Autodesk Inventor part; units mm, degrees
ref_plane "YZ Plane" through (0, 0, 0) normal (1, 0, 0) x (0, 1, 0)
ref_plane "XZ Plane" through (0, 0, 0) normal (0, 1, 0) x (-1, 0, 0)
ref_plane "XY Plane" through (0, 0, 0) normal (0, 0, 1) x (1, 0, 0)
sketch "Sketch2" plane through (0, 0, 0) normal (0, 0, 1) x (1, 0, 0)
  line L0 (0, 0) -> (44.45, 0)
  line L1 (44.45, 0) -> (44.45, 50.8)
  line L2 (44.45, 50.8) -> (0, 50.8)
  line L3 (0, 50.8) -> (0, 0)
  dimension "d0" = 50.8
  dimension "d1" = 44.45
extrude "Extrusion1" add sketch "Sketch2" along normal blind 25.4
sketch "Sketch3" plane through (0, 0, 25.4) normal (0, 0, 1) x (1, 0, 0)
  line L0 (2.54, 2.54) -> (20.32, 2.54)
  line L1 (20.32, 2.54) -> (20.32, 48.26)
  line L2 (20.32, 48.26) -> (2.54, 48.26)
  line L3 (2.54, 48.26) -> (2.54, 2.54)
  line L4 (0, 0) -> (44.45, 0)
  line L5 (0, 50.8) -> (0, 0)
  line L6 (44.45, 50.8) -> (0, 50.8)
  line L7 (21.59, 2.54) -> (41.91, 2.54)
  line L8 (41.91, 2.54) -> (41.91, 48.26)
  line L9 (41.91, 48.26) -> (21.59, 48.26)
  line L10 (21.59, 48.26) -> (21.59, 2.54)
  line L11 (44.45, 0) -> (44.45, 50.8)
  dimension "d4" = 2.54
  dimension "d5" = 2.54
  dimension "d6" = 2.54
  dimension "d7" = 20.32
  dimension "d8" = 2.54
  dimension "d9" = 2.54
  dimension "d10" = 2.54
  dimension "d11" = 22.86
extrude "Extrusion2" cut sketch "Sketch3" against normal blind 20.32 contours L3 L2 L1 L0 | L10 L9 L8 L7
sketch "Sketch4" plane through (0, 0, 0) normal (0, 0, -1) x (-1, 0, 0)
  circle A0 centre (-12.7, 17.78) radius 8.89
  line L0 (0, 50.8) -> (0, 0)
  line L1 (0, 0) -> (-44.45, 0)
  dimension "d14" = 17.78
  dimension "d17" = 12.7
  dimension "d18" = 17.78
extrude "Extrusion3" cut sketch "Sketch4" against normal blind 3.175
sketch "Sketch5" plane through (0, 0, 0) normal (0, 0, -1) x (-1, 0, 0)
  point P0 (0, 0)
sketch "Sketch6" plane through (12.7, 17.78, 3.175) normal (0, 0, -1) x (-1, 0, 0)
  circle A0 centre (0, 0) radius 8.89
  line L0 (0, 0) -> (-5.08, 0)
  line L1 (-5.08, 0) -> (-5.08, 12.7)
  line L2 (-5.08, 12.7) -> (0, 12.7)
  line L3 (0, 12.7) -> (0, 0)
  line L4 (0, 0) -> (5.08, 0)
  line L5 (5.08, 0) -> (5.08, 12.7)
  line L6 (5.08, 12.7) -> (0, 12.7)
  line L7 (0, 12.7) -> (0, 0)
  point P0 (12.7, -17.78)
  dimension "d21" = 12.7
  dimension "d22" = 5.08
  dimension "d23" = 5.08
extrude "Extrusion4" cut sketch "Sketch6" along normal blind 5.08 contours L5 L4 L3 A0 | A0 L3 L6 L5 | L1 L2 L3 A0 | A0 L3 L0 L1
sketch "Sketch7" plane through (0, 0, 3.175) normal (0, 0, -1) x (-1, 0, 0)
  point P0 (0, 0)
sketch "Sketch8" plane through (0, 0, 3.175) normal (0, 0, -1) x (-1, 0, 0)
  line L0 (-7.62, 25.0756) -> (-7.62, 30.48)
  line L1 (-17.78, 30.48) -> (-7.62, 30.48)
  line L2 (-7.62, 30.48) -> (-7.62, 26.67)
  line L3 (-7.62, 26.67) -> (-17.78, 26.67)
  line L4 (-17.78, 26.67) -> (-17.78, 30.48)
  point P0 (0, 0)
  dimension "d26" = 3.81
extrude "Extrusion5" cut sketch "Sketch8" against normal blind 2.54
sketch "Sketch14" plane through (41.91, 2.54, 25.4) normal (-1, 0, 0) x (0, 0, 1)
  line L0 (0, 0) -> (-20.32, 0)
  line L1 (0, 45.72) -> (-20.32, 45.72)
  line L2 (-12.7, 45.72) -> (-12.7, 43.18)
  line L3 (-12.7, 43.18) -> (-15.24, 45.72)
  line L4 (-12.7, 0) -> (-12.7, 2.54)
  line L5 (-12.7, 2.54) -> (-15.24, 0)
  point P0 (-25.4, -2.54)
  dimension "d52" = 45
  dimension "d53" = 2.54
  dimension "d54" = 2.54
  dimension "d55" = 45
  dimension "d56" = 5.08
  dimension "d57" = 5.08
extrude "Arduino Holder" add sketch "Sketch14" along normal blind 20.32
sketch "Sketch16" plane through (2.54, 2.54, 25.4) normal (0, 1, 0) x (1, 0, 0)
  line L0 (0, 12.7) -> (3.81, 12.7)
  line L1 (3.81, 12.7) -> (0, 16.51)
  line L2 (0, 0) -> (0, 20.32)
  line L3 (17.78, 5.08) -> (17.78, 20.32)
  line L4 (17.78, 16.51) -> (13.97, 12.7)
  line L5 (13.97, 12.7) -> (17.78, 12.7)
  line L6 (17.78, 20.32) -> (0, 20.32)
  point P0 (-2.54, 25.4)
  dimension "d60" = 45
  dimension "d61" = 3.81
  dimension "d62" = 3.81
  dimension "d64" = 45
  dimension "d144" = 7.62
  dimension "d145" = 7.62
extrude "Bluetooth Holder" add sketch "Sketch16" along normal blind 45.72
sketch "Sketch17" plane through (0, 0, 0) normal (-1, 0, 0) x (0, 0, 1)
  line L0 (0, 50.8) -> (25.4, 50.8)
  line L1 (0, 0) -> (5.08, 0)
  line L2 (5.08, 0) -> (5.08, 50.8)
  line L3 (5.08, 50.8) -> (0, 50.8)
  line L4 (0, 50.8) -> (0, 0)
  dimension "d68" = 5.08
extrude "Extrusion13" add sketch "Sketch17" along normal blind 5.08
sketch "Sketch18" plane through (0, 0, 5.08) normal (0, 0, 1) x (1, 0, 0)
  line L0 (0, 50.8) -> (0, 0)
  line L1 (0, 2.54) -> (-2.54, 2.54)
  line L2 (-2.54, 2.54) -> (-2.54, 48.26)
  line L3 (-2.54, 48.26) -> (0, 48.26)
  line L4 (0, 48.26) -> (0, 2.54)
  line L5 (0, 50.8) -> (-5.08, 50.8)
  line L6 (0, 0) -> (-5.08, 0)
  dimension "d71" = 2.54
  dimension "d72" = 2.54
  dimension "d73" = 2.54
extrude "Extrusion14" cut sketch "Sketch18" against normal blind 5.08
sketch "Sketch19" plane through (44.45, 0, 0) normal (1, 0, 0) x (0, 0, -1)
  line L0 (0, 50.8) -> (-25.4, 50.8)
  line L1 (0, 0) -> (-5.08, 0)
  line L2 (-5.08, 0) -> (-5.08, 50.8)
  line L3 (-5.08, 50.8) -> (0, 50.8)
  line L4 (0, 50.8) -> (0, 0)
  dimension "d76" = 5.08
extrude "Extrusion15" add sketch "Sketch19" along normal blind 5.08
sketch "Sketch21" plane through (44.45, 0, 5.08) normal (0, 0, 1) x (1, 0, 0)
  line L0 (0, 0) -> (0, 50.8)
  line L1 (0, 2.54) -> (2.54, 2.54)
  line L2 (2.54, 2.54) -> (2.54, 48.26)
  line L3 (2.54, 48.26) -> (0, 48.26)
  line L4 (0, 48.26) -> (0, 2.54)
  line L5 (0, 50.8) -> (5.08, 50.8)
  line L6 (0, 0) -> (5.08, 0)
  line L7 (5.08, 50.8) -> (5.08, 0)
  point P0 (-44.45, 0)
  dimension "d79" = 2.54
  dimension "d81" = 2.54
  dimension "d82" = 2.54
extrude "Extrusion16" cut sketch "Sketch21" against normal blind 5.08 contours L0 L3 L2 L1
sketch "Sketch28" plane through (0, 0, 25.4) normal (-1, 0, 0) x (0, 0, 1)
  line L0 (-20.32, 0) -> (0, 0)
  line L1 (0, 50.8) -> (-7.62, 50.8)
  line L2 (-7.62, 50.8) -> (-7.62, 0)
  line L3 (-7.62, 0) -> (0, 0)
  line L4 (0, 0) -> (0, 50.8)
  point P0 (-25.4, 0)
  dimension "d141" = 7.62
extrude "Height Reduce" cut sketch "Sketch28" against normal blind 50.8
sketch "Sketch30" plane through (0, 0, 5.08) normal (0, 0, 1) x (1, 0, 0)
  line L0 (22.86, 5.08) -> (40.64, 5.08)
  line L1 (40.64, 5.08) -> (40.64, 26.67)
  line L2 (40.64, 26.67) -> (22.86, 26.67)
  line L3 (22.86, 26.67) -> (22.86, 5.08)
  line L4 (21.59, 2.54) -> (21.59, 48.26)
  line L5 (41.91, 48.26) -> (41.91, 2.54)
  line L6 (41.91, 2.54) -> (21.59, 2.54)
  point P0 (0, 0)
  point P1 (24.13, 12.7)
  point P2 (44.45, 30.48)
  dimension "d146" = 1.27
  dimension "d147" = 1.27
  dimension "d148" = 21.59
  dimension "d149" = 2.54
  dimension "d150" = 17.78
extrude "Extrusion27" cut sketch "Sketch30" against normal blind 2.54
sketch "Sketch31" plane through (0, 0, 5.08) normal (0, 0, 1) x (1, 0, 0)
  line L0 (21.59, 2.54) -> (21.59, 48.26)
  line L1 (41.91, 48.26) -> (41.91, 2.54)
  line L2 (21.59, 45.72) -> (41.91, 45.72)
  line L3 (41.91, 45.72) -> (41.91, 29.21)
  line L4 (41.91, 29.21) -> (21.59, 29.21)
  line L5 (21.59, 29.21) -> (21.59, 45.72)
  line L6 (21.59, 48.26) -> (41.91, 48.26)
  line L7 (21.59, 40.64) -> (29.21, 40.64)
  line L8 (29.21, 40.64) -> (29.21, 34.29)
  line L9 (29.21, 34.29) -> (21.59, 34.29)
  line L10 (21.59, 34.29) -> (21.59, 40.64)
  line L11 (41.91, 45.72) -> (36.83, 45.72)
  line L12 (36.83, 45.72) -> (36.83, 29.21)
  line L13 (36.83, 29.21) -> (41.91, 29.21)
  line L14 (41.91, 29.21) -> (41.91, 45.72)
  point P0 (0, 0)
  point P1 (24.13, 33.02)
  dimension "d157" = 2.54
  dimension "d158" = 16.51
  dimension "d159" = 5.08
  dimension "d160" = 6.35
  dimension "d161" = 7.62
  dimension "d162" = 5.08
  dimension "d163" = 5.08
extrude "Extrusion28" cut sketch "Sketch31" against normal blind 25.4 contours L0 L7 L8 L9
extrude "Extrusion29" cut sketch "Sketch31" against normal blind 2.54 contours L12 L2 L1 L4
extrude "Extrusion30" cut sketch "Sketch31" against normal blind 1.27 contours L0 L9 L8 L7 L2 L12 L4
sketch "Sketch33" plane through (44.45, 2.54, 0) normal (1, 0, 0) x (0, 0, -1)
  line L0 (-5.08, 48.26) -> (-17.78, 48.26)
  line L1 (-17.78, -2.54) -> (-15.24, -2.54)
  line L2 (-15.24, -2.54) -> (-15.24, 48.26)
  line L3 (-15.24, 48.26) -> (-17.78, 48.26)
  line L4 (-17.78, 48.26) -> (-17.78, -2.54)
  point P0 (0, -2.54)
  dimension "d194" = 2.54
extrude "Extrusion33" add sketch "Sketch33" along normal blind 2.54
sketch "Sketch35" plane through (0, 2.54, 0) normal (-1, 0, 0) x (0, 0, 1)
  line L0 (5.08, 48.26) -> (17.78, 48.26)
  line L1 (17.78, -2.54) -> (15.24, -2.54)
  line L2 (15.24, -2.54) -> (15.24, 48.26)
  line L3 (15.24, 48.26) -> (17.78, 48.26)
  line L4 (17.78, 48.26) -> (17.78, -2.54)
  point P0 (0, -2.54)
  dimension "d197" = 2.54
extrude "Extrusion34" add sketch "Sketch35" along normal blind 2.54
sketch "Sketch36" plane through (-5.08, 0, 5.08) normal (0, -1, 0) x (1, 0, 0)
  line L0 (2.54, 12.7) -> (5.08, 10.16)
  line L1 (5.08, 10.16) -> (2.54, 10.16)
  line L2 (5.08, 10.16) -> (2.54, 10.16)
  line L3 (2.54, 10.16) -> (2.54, 12.7)
  line L4 (49.53, 10.16) -> (52.07, 12.7)
  line L5 (52.07, 12.7) -> (52.07, 10.16)
  line L6 (52.07, 10.16) -> (49.53, 10.16)
  point P0 (5.08, -5.08)
extrude "Extrusion35" cut sketch "Sketch36" against normal blind 50.8
sketch "Sketch37" plane through (-5.08, 50.8, 5.08) normal (0, 1, 0) x (1, 0, 0)
  line L0 (52.07, -12.7) -> (2.54, -12.7)
  line L1 (41.91, -12.7) -> (31.75, -12.7)
  line L2 (31.75, -12.7) -> (31.75, -8.89)
  line L3 (31.75, -8.89) -> (41.91, -8.89)
  line L4 (41.91, -8.89) -> (41.91, -12.7)
  line L5 (26.67, -12.7) -> (26.67, -7.62)
  line L6 (46.99, -12.7) -> (46.99, -7.62)
  point P0 (5.08, 5.08)
  dimension "d202" = 3.81
  dimension "d203" = 10.16
  dimension "d204" = 5.08
  dimension "d205" = 5.08
extrude "Extrusion36" cut sketch "Sketch37" against normal blind 2.54
sketch "Sketch39" plane through (21.59, 2.54, 12.7) normal (1, 0, 0) x (0, 0, -1)
  line L0 (7.62, 0) -> (2.54, 5.08)
  line L1 (2.54, 5.08) -> (-5.08, 5.08)
  line L2 (-5.08, 45.72) -> (-5.08, 0)
  line L3 (-5.08, 5.08) -> (-5.08, 40.64)
  line L4 (-5.08, 40.64) -> (2.54, 40.64)
  line L5 (2.54, 40.64) -> (7.62, 45.72)
  line L6 (7.62, 45.72) -> (7.62, 0)
  line L7 (7.62, 2.54) -> (10.16, 2.54)
  point P0 (12.7, -2.54)
  dimension "d224" = 45
  dimension "d225" = 45
  dimension "d226" = 5.08
extrude "Extrusion38" cut sketch "Sketch39" against normal blind 5.08
properties part number "nano_enclosure_v3_1"
The model under review builds one solid part; all positions refer to its coordinate system, in mm. A direction names the side the tool comes from. Coordinates: 2 decimals unless noted, no trailing zeros. Loops run counter-clockwise (first coordinate to the right, second up) from the corner with the lowest first, then second, coordinate; pieces in that order, holes last. Notation, with made-up numbers: M 8.25,-30.5 L 29.25,-30.5 A25 cw 29.25,3.5 Z; hole C -24,10 d3. An arc over 180 degrees is marked long. Put each result on its own line as item: value. Start each with the question number.
Q1. Add section D-D (y = 35.5). Write out the cut boundary in (x, z).
Q2. The part is to be moulded in two halves that separate along Y. For faces 1 (the flat face through (32, 4, 12.7)), 2 (the flat face through (23, 0, 9)), 3 (the flat face through (22, 26, 0)), say which applies: +Y half, -Y half, draft (parallel to the pull), parting line (faces both ways), or undercut.
Q3. Add section B-B (x = 12.7). Write out the cut boundary in (y, z) (3 decimals).
Q4. For faces 4 (the flat face through (20.9, 45.68, 7.66)), 5 (the flat face through (-1, 48.26, 3)), 6 (the flat face through (32, 47, 12.7)), 7 (the flat face through (13, 30.48, 3)), list the 3-axis set-ups (+Z, -Z, +X, -X, +Y, -Y) from which the entire face can be reached by the end or side of a thin tool; tool diameter is ignored.
Q5. Clearance check with flat-ended pins moving along their axes: pin 1 (6 mm diameter, centred on x = 39.5, z = 13, fed in from -Y); pin 2 (2.5 mm diameter, centred on y = 46.5, z = 13.5, fed in from +X); pin 3 (3 mm diameter, centred on y = 8, z = 15, fed in from +X); pin 4 (3 mm diameter, centred on x = 20.5, y = 18, fed in from +Z). State where each tip first meets the part, or that it passes through.
Q6. Add section A-A (y = 17.78). Count the separate pieces of the cut face and the enclosed holes in it, and give its area (3 significant figures).
Q7. Add section C-C (z = 12). Write out the cut boundary in (x, y), and give its area (3 significant figures).
Q8. Wall thickness on line 1 (X direction, y = 17.78, z = 1.8); line 2 (X direction, y = 38, z = 1); line 3 (X direction, y = 3.5, z = 2): over which ranges is each line inside the solid? List them lowest first.
Answers:
1. outline: M -5.08,0 L -2.54,0 L -2.54,5.08 L -5.08,5.08 Z; M -2.54,17.78 L 0,15.24 L 0,0 L 21.59,0 L 21.59,5.08 L 2.54,5.08 L 2.54,8.89 L 6.35,12.7 L 2.54,12.7 L 2.54,17.78 Z; M 29.21,0 L 44.45,0 L 44.45,15.24 L 46.99,17.78 L 41.91,17.78 L 41.91,2.54 L 36.83,2.54 L 36.83,3.81 L 29.21,3.81 Z; M 46.99,0 L 49.53,0 L 49.53,5.08 L 46.99,5.08 Z
2. face 1: undercut
2. face 2: -Y half
2. face 3: draft
3. outline: M 0,0 L 8.89,0 L 8.89,3.175 L 26.67,3.175 L 26.67,5.08 L 2.54,5.08 L 2.54,17.78 L 0,17.78 Z; M 30.48,0 L 50.8,0 L 50.8,17.78 L 48.26,17.78 L 48.26,5.08 L 30.48,5.08 Z
4. face 4: none
4. face 5: -Z
4. face 6: +Z
4. face 7: +Z, -Z
5. pin 1: stops at y = 0
5. pin 2: stops at x = 44.45
5. pin 3: stops at x = 45.71
5. pin 4: stops at z = 5.08
6. separate pieces: 3
6. enclosed holes: 0
6. area: 228 mm^2
7. outline: M 0,0 L 44.45,0 L 44.45,50.8 L 0,50.8 Z; hole M 5.65,2.54 L 17.21,2.54 L 17.21,7.62 L 21.59,7.62 L 21.59,4.38 L 41.91,4.38 L 41.91,46.42 L 21.59,46.42 L 21.59,43.18 L 17.21,43.18 L 17.21,48.26 L 5.65,48.26 Z
7. area: 720 mm^2
8. line 1: x = -5.08 to -2.54, 0 to 3.81, 21.59 to 44.45, 46.99 to 49.53
8. line 2: x = -5.08 to -2.54, 0 to 21.59, 29.21 to 44.45, 46.99 to 49.53
8. line 3: x = -5.08 to -2.54, 0 to 44.45, 46.99 to 49.53
